Geometry check sheet. Reference: the model listing, model coordinates, mm. Face numbers are marked on the shaded views. A direction names the side the tool comes from. Round coordinates to 2 decimals unless told otherwise and drop trailing zeros. Order: outer loops, then holes, each group sorted by start corner. A loop starts at its lowest first (then second) coordinate and runs counter-clockwise, first axis right, second up. Notation, with made-up numbers: (54.5, 87.5) - (62.5, 87.5) arc R21 cw to (62.5, 125.5) - close; hole circle Ø4 at (66.25, 4.25). An arc over 180 degrees is marked (long way). Return JSON: item names as keys, results as strings. Group by question number.
Q1. Sectioned sample at B-B, the plane z = -10. Record the cut outline in (x, y) (3 decimals).
Q2. Sectioned sample at D-D, the plane z = 0. Record the cut outline in (x, y).
Q3. Draft check along X on the marked faces 1, 2 and 3. Enter one of: pulls with the +X half, pulls with the -X half, needs draft (parallel to the pull), parting line crosses it, or undercut.
Q4. Tool access check on the marked faces 4, 5, 6, 7 and 8. Record the directions out of +Z, -Z, +X, -X, +Y, -Y that give a thin tool (end or side, any length) a straight path to the whole face; none if there is none.
Q5. Gauge pin test, flat ends, axial feed: pin 1 Ø6 at (x, z) = (-5, -26.5) entering from +Y; pin 2 Ø5 at (x, y) = (-17, 0) entering from -Z; pin 3 Ø8 at (x, z) = (11.5, -9) entering from -Y; pin 4 Ø11 at (y, z) = (-25, -11.5) entering from +X. Record the tip position at first contact, or that the pin passes through.
Q6. Material ranges on line 1 along X through (y, z) = (-5, -23); line 2 along X through (y, z) = (4, -6.5); line 3 along Y through (x, z) = (-19.55, -10), recorded low to high.
Q7. Sectioned sample at A-A, the plane x = 8. Record the cut outline in (y, z).
Q8. Sectioned sample at C-C, the plane y = -5. Record the cut outline in (x, z).
```python
from build123d import *

# Parameters (mm, degrees)
BOSS_EXTRUDE1_DEPTH                                 = 20
SKETCH2_W                                           = 53
SKETCH2_H                                           = 20
BOSS_EXTRUDE2_DEPTH                                 = 8
SKETCH11_W                                          = 60
SKETCH11_H                                          = 20
BOSS_EXTRUDE3_DEPTH                                 = 10
M3_TAPPED_HOLE1_D                                   = 2.5
CSK_FOR_M4_COUNTERSUNK_FLAT_HEAD_SCREW1_D           = 4.5
CSK_FOR_M4_COUNTERSUNK_FLAT_HEAD_SCREW1_CSINK_D     = 9.4
CSK_FOR_M4_COUNTERSUNK_FLAT_HEAD_SCREW1_CSINK_ANGLE = 90
CHAMFER1_SIZE                                       = 15
CBORE_FOR_M5_HEX_SOCKET_HEAD_CAP_SCR_2_COUNT        = 2
CBORE_FOR_M5_HEX_SOCKET_HEAD_CAP_SCR_2_PITCH        = 20
CBORE_FOR_M5_HEX_SOCKET_HEAD_CAP_SCR_3_COUNT        = 2
CBORE_FOR_M5_HEX_SOCKET_HEAD_CAP_SCR_3_PITCH        = 40


with BuildPart() as part:
    # Sketch1 → Boss-Extrude1 (new, symmetric)
    with BuildSketch(Plane.XY):
        Polygon((-23.5, 11.5), (-23.5, -3.5), (23.5, -3.5), (23.5, 11.5), (26.5, 11.5), (26.5, -11.5), (-26.5, -11.5), (-26.5, 11.5), align=None)
    extrude(amount=BOSS_EXTRUDE1_DEPTH, both=True)

    # Sketch2 → Boss-Extrude2 (add)
    with BuildSketch(Plane(origin=(0, -3.5, 0), x_dir=(1, 0, 0), z_dir=(0, 1, 0))):
        with Locations((0, 30)):
            Rectangle(SKETCH2_W, SKETCH2_H)
    extrude(amount=-BOSS_EXTRUDE2_DEPTH)

    # Sketch11 → Boss-Extrude3 (add)
    with BuildSketch(Plane(origin=(-26.5, 0, 0), x_dir=(0, 0, -1), z_dir=(1, 0, 0))):
        with Locations((10, -21.5)):
            Rectangle(SKETCH11_W, SKETCH11_H)
    extrude(amount=BOSS_EXTRUDE3_DEPTH)

    # M3 Tapped Hole1 (through all)
    with Locations(Plane(origin=(0, -3.5, 0), x_dir=(1, 0, 0), z_dir=(0, 1, 0))):
        with Locations((0, 35), (-5, 23), (5, 23)):
            Hole(M3_TAPPED_HOLE1_D / 2)

    # CSK for M4 Countersunk Flat Head Screw1 (through all)
    with Locations(Plane(origin=(0, -3.5, 0), x_dir=(1, 0, 0), z_dir=(0, 1, 0))):
        with Locations((-8, 0), (8, 0)):
            CounterSinkHole(CSK_FOR_M4_COUNTERSUNK_FLAT_HEAD_SCREW1_D / 2, CSK_FOR_M4_COUNTERSUNK_FLAT_HEAD_SCREW1_CSINK_D / 2, counter_sink_angle=CSK_FOR_M4_COUNTERSUNK_FLAT_HEAD_SCREW1_CSINK_ANGLE)

    # Chamfer1
    chamfer1_edges = [part.edges().sort_by_distance(p)[0] for p in [
        (-25, -3.5, -20),
        (25, -3.5, -20),
    ]]
    chamfer(chamfer1_edges, length=CHAMFER1_SIZE - 0.0001)  # a hair under: the kernel refuses the full size

    # Sketch14 → CBORE for M5 Hex Socket Head Cap Screw1 (revolve, cut)
    with BuildSketch(Plane(origin=(-16.5, -23.5, -30), x_dir=(0, 0, -1), z_dir=(0, 1, 0))):
        Polygon((0, 0), (0, 10), (2.775, 10), (2.75, 9.975), (2.75, 5.4), (5, 5.4), (5, 0.025), (5.025, 0), align=None)
    cbore_for_m5_hex_socket_head_cap_screw1 = revolve(axis=Axis((-10.15, -23.5, -30), (-1, 0, 0)), mode=Mode.SUBTRACT)

    # CBORE for M5 Hex Socket Head Cap Scr 2: CBORE for M5 Hex Socket Head Cap Screw1 ×2
    with Locations(*[(0, 0, i * CBORE_FOR_M5_HEX_SOCKET_HEAD_CAP_SCR_2_PITCH) for i in range(1, CBORE_FOR_M5_HEX_SOCKET_HEAD_CAP_SCR_2_COUNT)]):
        add(cbore_for_m5_hex_socket_head_cap_screw1, mode=Mode.SUBTRACT)

    # CBORE for M5 Hex Socket Head Cap Scr 3: CBORE for M5 Hex Socket Head Cap Screw1 ×2
    with Locations(*[(0, 0, i * CBORE_FOR_M5_HEX_SOCKET_HEAD_CAP_SCR_3_PITCH) for i in range(1, CBORE_FOR_M5_HEX_SOCKET_HEAD_CAP_SCR_3_COUNT)]):
        add(cbore_for_m5_hex_socket_head_cap_screw1, mode=Mode.SUBTRACT)


solid = part.part
```
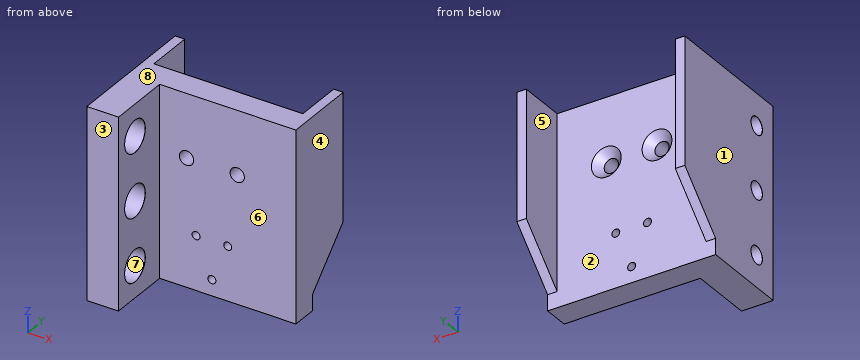
Reply:
{
 "1": {"outline": "(-26.5, -31.5) - (-16.5, -31.5) - (-16.5, -28.525) - (-16.525, -28.5) - (-21.9, -28.5) - (-21.9, -26.25) - (-26.475, -26.25) - (-26.5, -26.275) - close; (-26.5, -20.725) - (-26.475, -20.75) - (-21.9, -20.75) - (-21.9, -18.5) - (-16.525, -18.5) - (-16.5, -18.475) - (-16.5, -11.5) - (26.5, -11.5) - (26.5, 11.5) - (23.5, 11.5) - (23.5, -3.5) - (-23.5, -3.5) - (-23.5, 11.5) - (-26.5, 11.5) - close"},
 "2": {"outline": "(-26.5, -31.5) - (-16.5, -31.5) - (-16.5, -11.5) - (-10.25, -11.5) - (-10.25, -5.95) - (-12.7, -3.5) - (-23.5, -3.5) - (-23.5, 11.5) - (-26.5, 11.5) - close; (-5.75, -11.5) - (5.75, -11.5) - (5.75, -5.95) - (3.3, -3.5) - (-3.3, -3.5) - (-5.75, -5.95) - close; (10.25, -11.5) - (26.5, -11.5) - (26.5, 11.5) - (23.5, 11.5) - (23.5, -3.5) - (12.7, -3.5) - (10.25, -5.95) - close"},
 "3": {"face 1": "pulls with the -X half", "face 2": "undercut", "face 3": "needs draft"},
 "4": {"face 4": "+Z, -Z, +X, +Y, -Y", "face 5": "+Z, -Z, +Y", "face 6": "+Z, -Z, +X, -Y", "face 7": "+X", "face 8": "+Z, +X, -X, +Y, -Y"},
 "5": {"pin 1": "y = -3.5", "pin 2": "through", "pin 3": "y = -11.5", "pin 4": "x = -16.5"},
 "6": {"line 1": "-26.5 to -6.25, -3.75 to 3.75, 6.25 to 26.5", "line 2": "-26.5 to -23.5, 23.5 to 26.5", "line 3": "-31.5 to -28.5, -18.5 to -3.5"},
 "7": {"outline": "(-11.5, -40) - (-3.5, -40) - (-3.5, -4.7) - (-5.95, -2.25) - (-11.5, -2.25) - close; (-11.5, 2.25) - (-5.95, 2.25) - (-3.5, 4.7) - (-3.5, 20) - (-11.5, 20) - close"},
 "8": {"outline": "(-26.5, -40) - (26.5, -40) - (26.5, 20) - (-26.5, 20) - close; hole circle Ø6.4 at (-8, 0); hole circle Ø2.5 at (-5, -23); hole circle Ø2.5 at (0, -35); hole circle Ø2.5 at (5, -23); hole circle Ø6.4 at (8, 0)"}
}
